The model under review builds one solid part; all positions refer to its coordinate system, in mm. Round coordinates to 2 decimals unless told otherwise and drop trailing zeros. Write each loop counter-clockwise with the first axis right and the second up, starting at its lowest first coordinate (ties: lowest second). Pieces come first, ordered by that corner, then holes. Notation, with made-up numbers: (-26, -4.75) - (-21, -4.75) arc R20 cw to (-21, 10.25) - close; hole circle Ø8 at (47, -17.75). An arc over 180 degrees is marked (long way). Return JSON: item names as keys, results as strings.
from build123d import *

# Parameters (mm, degrees)
SKETCH1_W                 = 15.875
SKETCH1_H                 = 9.525
BOSS_EXTRUDE1_DEPTH       = 1.5875
F_4_CLEARANCE_HOLE1_D     = 2.9464
F_4_CLEARANCE_HOLE1_DEPTH = 1.5875


with BuildPart() as part:
    # Sketch1 → Boss-Extrude1 (new body)
    with BuildSketch(Plane.XY):
        Rectangle(SKETCH1_W, SKETCH1_H)
    extrude(amount=BOSS_EXTRUDE1_DEPTH)

    # #4 Clearance Hole1
    with Locations(Plane.XY.offset(1.5875)):
        with Locations((-5.0673, 0), (5.0673, 0)):
            Hole(F_4_CLEARANCE_HOLE1_D / 2, depth=F_4_CLEARANCE_HOLE1_DEPTH)


solid = part.part
(1) Mouldability with a two-part tool opening along Y and no side actions: class faces 1 (the cylindrical face through (-6.43, -0.56, 0.78)), 2 (the cylindrical face through (6.54, 0.06, 0.78)), 3 (the flat face through (0, -4.762, 1)), 4 (the flat face through (7.938, 0, 1)) as released by +Y, released by -Y, zero draft, split by the parting line, or undercut.
Filled in:
{"face 1": "undercut", "face 2": "undercut", "face 3": "released by -Y", "face 4": "zero draft"}
(2) Add section B-B (z = 0.15). Write out the cut boundary in (x, y).
Filled in:
{"outline": "(-7.94, -4.76) - (7.94, -4.76) - (7.94, 4.76) - (-7.94, 4.76) - close; hole circle Ø2.95 at (-5.07, 0); hole circle Ø2.95 at (5.07, 0)"}
(3) Add section A-A (y = 0). Write out the cut boundary in (x, z), plus the area to 3 significant figures.
Filled in:
{"outline": "(-7.94, 0) - (-6.54, 0) - (-6.54, 1.59) - (-7.94, 1.59) - close; (-3.59, 0) - (3.59, 0) - (3.59, 1.59) - (-3.59, 1.59) - close; (6.54, 0) - (7.94, 0) - (7.94, 1.59) - (6.54, 1.59) - close", "area": "15.8 mm2"}
(4) Add section C-C (x = 5.5). Write out the cut boundary in (y, z), plus the area to 3 significant figures.
Filled in:
{"outline": "(-4.76, 0) - (-1.41, 0) - (-1.41, 1.59) - (-4.76, 1.59) - close; (1.41, 0) - (4.76, 0) - (4.76, 1.59) - (1.41, 1.59) - close", "area": "10.6 mm2"}
(5) Wall thickness on line 1 (X direction, y = -0.25, z = 0.15); line 2 (X direction, y = -0.5, z = 0.3); line 3 (Y direction, x = -5.5, z = 1.35): over which ranges is each line inside the solid? List them lowest first.
Filled in:
{"line 1": "x = -7.94 to -6.52, -3.62 to 3.62, 6.52 to 7.94", "line 2": "x = -7.94 to -6.45, -3.68 to 3.68, 6.45 to 7.94", "line 3": "y = -4.76 to -1.41, 1.41 to 4.76"}
(6) Add section D-D (y = 1.25). Write out the cut boundary in (x, z), plus the area to 3 significant figures.
Filled in:
{"outline": "(-7.94, 0) - (-5.85, 0) - (-5.85, 1.59) - (-7.94, 1.59) - close; (-4.29, 0) - (4.29, 0) - (4.29, 1.59) - (-4.29, 1.59) - close; (5.85, 0) - (7.94, 0) - (7.94, 1.59) - (5.85, 1.59) - close", "area": "20.3 mm2"}
